Design review of the part shown in the three views and the two pictorial views. Dimensions are in mm from the part's minimum x, y and z. A direction names the side the tool comes from. Give positions to 0.01 mm unless a question says otherwise; leave off trailing zeros. Order: outer loops, then holes, each group sorted by start corner. A loop starts at its lowest first (then second) coordinate and runs counter-clockwise, first axis right, second up. Notation, with made-up numbers: (65, 17.5) -> (83, 17.5) arc R4 cw to (83, 22.5) -> close; hole circle Ø8 at (41.5, 66.5). An arc over 180 degrees is marked (long way). Answer in a Markdown table with one row per item. Add a question column.
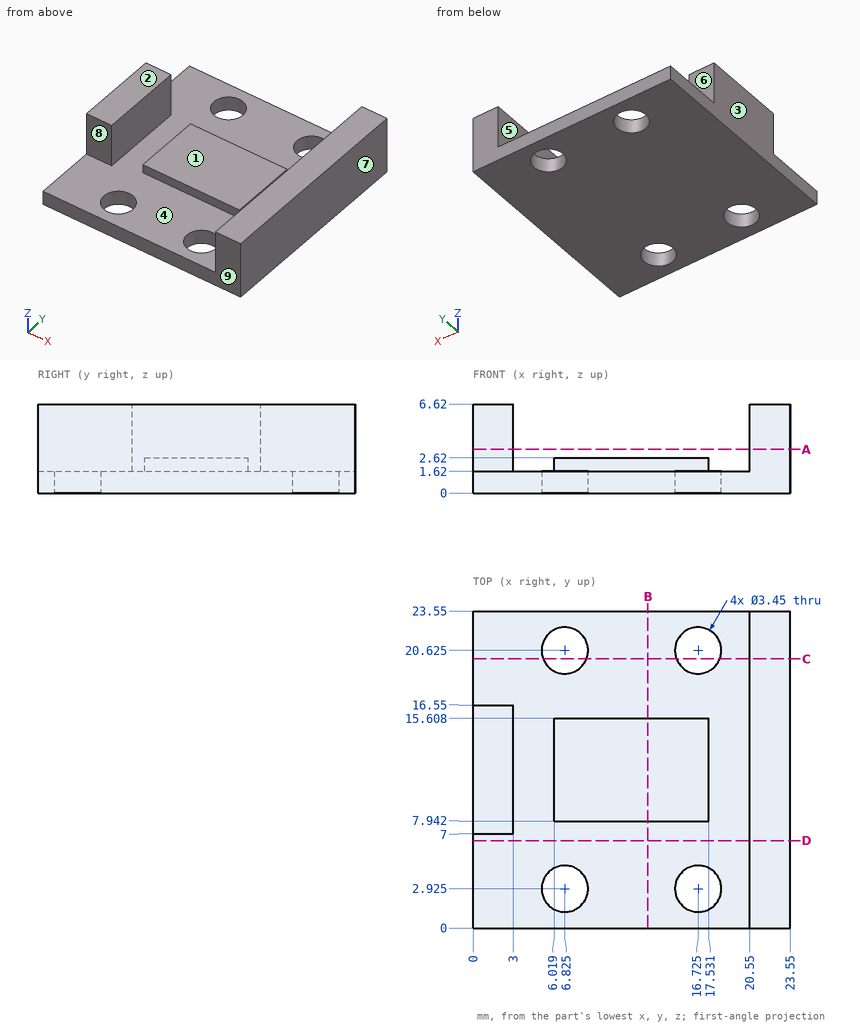
1) Clearance check with flat-ended pins moving along their axes: P1, Ø3, axis at x = 6.825, y = 20.625, coming from the +Z side; P2, Ø2.5, axis at x = 1, z = 5, coming from the +Y side; P3, Ø3.5, axis at x = 1.5, z = 5.5, coming from the -Y side; P4, Ø4.5, axis at x = 16.725, y = 2.925, coming from the +Z side. State where each tip first meets the part, or that it passes through.
2) Add section D-D, the plane y = 6.5. Write out the cut boundary in (x, z).
3) Add section C-C, the plane y = 20. Write out the cut boundary in (x, z).
4) Add section A-A, the plane z = 3.25. Write out the cut boundary in (x, y).
5) Machinability: for the marked faces 5, 6, 7, 8 and 9, which of the approach directions +Z, -Z, +X, -X, +Y, -Y give a long, thin tool a straight path to every point of the face, cutting with its end or side? Answer none if there is none.
6) Add section B-B, the plane x = 13. Write out the cut boundary in (y, z).
7) For L1, parallel to X at y = 9.25, z = 4; L2, parallel to X at y = 20.75, z = 2.75; L3, parallel to Z at x = 4.5, y = 2.5, list the stretches that pass through material, from the lowest coordinate up.
8) Mouldability with a two-part tool opening along X and no side actions: class the marked faces 1, 2, 3 and 4 as +X half, -X half, draft (parallel to the pull), parting line (faces both ways), or undercut.
Verdict:
| question | item | result |
|---|---|---|
| 1 | P1 | passes through |
| 1 | P2 | stops at y = 16.55 |
| 1 | P3 | stops at y = 7 |
| 1 | P4 | stops at z = 1.62 |
| 2 | outline | (0, 0) -> (23.55, 0) -> (23.55, 6.62) -> (20.55, 6.62) -> (20.55, 1.62) -> (0, 1.62) -> close |
| 3 | outline | (0, 0) -> (5.22, 0) -> (5.22, 1.62) -> (0, 1.62) -> close; (8.43, 0) -> (15.12, 0) -> (15.12, 1.62) -> (8.43, 1.62) -> close; (18.33, 0) -> (23.55, 0) -> (23.55, 6.62) -> (20.55, 6.62) -> (20.55, 1.62) -> (18.33, 1.62) -> close |
| 4 | outline | (0, 7) -> (3, 7) -> (3, 16.55) -> (0, 16.55) -> close; (20.55, 0) -> (23.55, 0) -> (23.55, 23.55) -> (20.55, 23.55) -> close |
| 5 | face 5 | +Z, +Y, -Y |
| 5 | face 6 | +Z, -X, +Y |
| 5 | face 7 | +Z, -Z, +X, +Y, -Y |
| 5 | face 8 | +Z, -X, -Y |
| 5 | face 9 | +Z, -Z, +X, -X, -Y |
| 6 | outline | (0, 0) -> (23.55, 0) -> (23.55, 1.62) -> (15.61, 1.62) -> (15.61, 2.62) -> (7.94, 2.62) -> (7.94, 1.62) -> (0, 1.62) -> close |
| 7 | L1 | x = 0 to 3, 20.55 to 23.55 |
| 7 | L2 | x = 20.55 to 23.55 |
| 7 | L3 | z = 0 to 1.62 |
| 8 | face 1 | undercut |
| 8 | face 2 | draft |
| 8 | face 3 | -X half |
| 8 | face 4 | undercut |
